Geometry: see drawing. Coordinates: mm, zero at the bounding-box minimum. A direction names the side the tool comes from. Round coordinates to 2 decimals unless told otherwise and drop trailing zeros. Loops run counter-clockwise (first coordinate to the right, second up) from the corner with the lowest first, then second, coordinate; pieces in that order, holes last. Notation, with made-up numbers: (12, 75.25) - (32, 75.25) arc R20 cw to (32, 86.25) - close; hole circle Ø2 at (47.25, -8.75). An arc over 180 degrees is marked (long way). Write item = value, one per line. Start each with the question number.
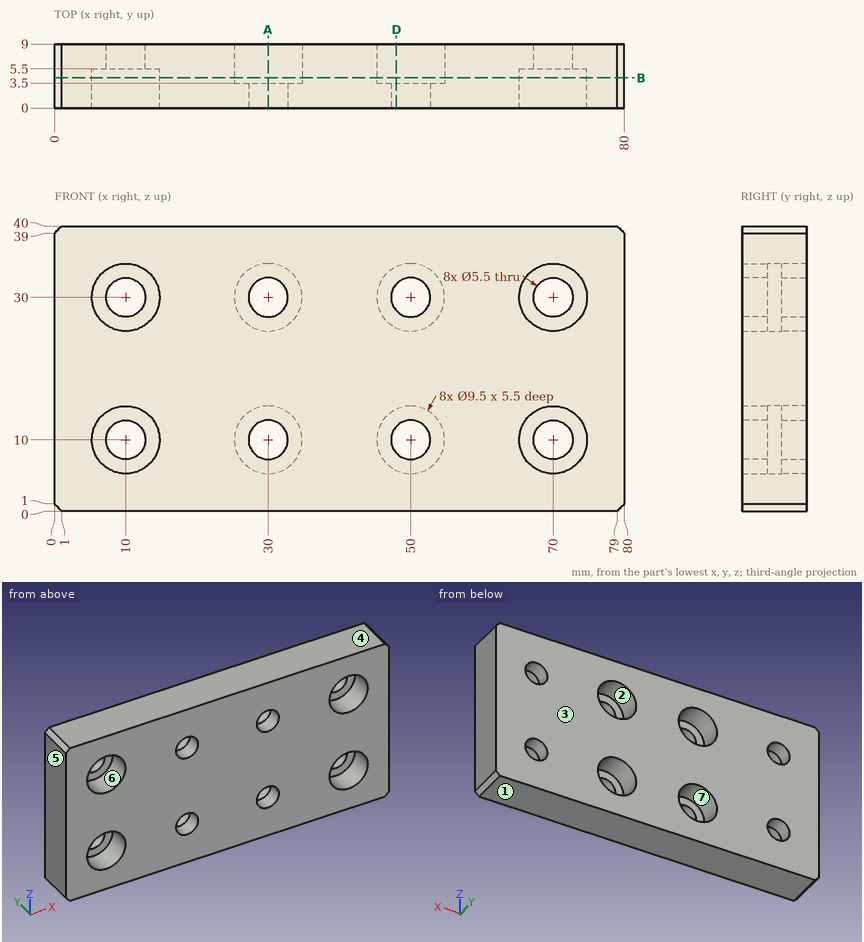
(1) Cut plane A-A (x = 30). Output: boundary loops of the cut face in (y, z), and give its area (3 significant figures).
(2) Access query for the marked faces 5, 6 and 7. Directions: +Z, -Z, +X, -X, +Y, -Y. A direction counts if a zero-diameter tool reaches every point of the face in a straight line with its end or side. Return the directions, or none.
(3) Cut plane D-D (x = 48). Output: boundary loops of the cut face in (y, z).
(4) Mould query, pull axis Z, two halves, no side actions, for the marked faces 1, 2, 3 and 4. Classes: +Z half, -Z half, draft (parallel to the pull), parting line (faces both ways), or undercut.
(5) Cut plane B-B (y = 4.25). State how many separate pieces and enclosed holes the cut face has, and give its area (3 significant figures).
(6) Material intervals for line 1 along Z through (x, y) = (10, 3.45); line 2 along Z through (x, y) = (70, 7.25); line 3 along X through (y, z) = (0.7, 30), sorted ascending. Write a range as from..to.
(7) Pin query (flat end, axial travel): P1, Ø5, axis at x = 50, z = 10, coming from the +Y side; P2, Ø5, axis at x = 31.5, z = 9.5, coming from the +Y side; P3, Ø7, axis at x = 70, z = 10, coming from the -Y side. Return the tip coordinate at first contact, or that it passes through.
Solution:
q1.outline = (0, 0) - (9, 0) - (9, 5.25) - (3.5, 5.25) - (3.5, 7.25) - (0, 7.25) - close; (0, 12.75) - (3.5, 12.75) - (3.5, 14.75) - (9, 14.75) - (9, 25.25) - (3.5, 25.25) - (3.5, 27.25) - (0, 27.25) - close; (0, 32.75) - (3.5, 32.75) - (3.5, 34.75) - (9, 34.75) - (9, 40) - (0, 40) - close
q1.area = 217 mm^2
q2.face_5 = +Z, -Z, -X, +Y, -Y
q2.face_6 = -Y
q2.face_7 = +Y
q3.outline = (0, 0) - (9, 0) - (9, 5.69) - (3.5, 5.69) - (3.5, 8.11) - (0, 8.11) - close; (0, 11.89) - (3.5, 11.89) - (3.5, 14.31) - (9, 14.31) - (9, 25.69) - (3.5, 25.69) - (3.5, 28.11) - (0, 28.11) - close; (0, 31.89) - (3.5, 31.89) - (3.5, 34.31) - (9, 34.31) - (9, 40) - (0, 40) - close
q4.face_1 = -Z half
q4.face_2 = undercut
q4.face_3 = draft
q4.face_4 = +Z half
q5.separate_pieces = 1
q5.enclosed_holes = 8
q5.area = 2,630 mm^2
q6.line_1 = 0..5.25, 14.75..25.25, 34.75..40
q6.line_2 = 0..7.25, 12.75..27.25, 32.75..40
q6.line_3 = 0..5.25, 14.75..27.25, 32.75..47.25, 52.75..65.25, 74.75..80
q7.P1 = through
q7.P2 = 3.5
q7.P3 = 5.5
